```python
from build123d import *

# Parameters (mm, degrees)
ESQUISSE2_W             = 154.6
ESQUISSE2_H             = 3
BOSS_EXTRU_1_DEPTH      = 64.27
ESQUISSE3_R             = 2.5
ENL_V_MAT_EXTRU_1_DEPTH = 101.761443216
ENL_V_MAT_EXTRU_2_DEPTH = 101.761443216


with BuildPart() as part:
    # Esquisse2 → Boss.-Extru.1 (new body)
    with BuildSketch(Plane(origin=(0, 0, 0), x_dir=(1, 0, 0), z_dir=(0, 1, 0))):
        with Locations((-0.245054897, 0)):
            Rectangle(ESQUISSE2_W, ESQUISSE2_H)
    extrude(amount=BOSS_EXTRU_1_DEPTH)

    # Esquisse3 → Enlèv. mat.-Extru.1 (cut, through all)
    with BuildSketch(Plane.XY.offset(1.5)):
        with Locations((-67.545054897, 16.0675)):
            Circle(ESQUISSE3_R)
        with Locations((-67.545054897, 48.2025)):
            Circle(ESQUISSE3_R)
        with Locations((67.054945103, 48.2025)):
            Circle(ESQUISSE3_R)
        with Locations((67.054945103, 16.0675)):
            Circle(ESQUISSE3_R)
    extrude(amount=-ENL_V_MAT_EXTRU_1_DEPTH, mode=Mode.SUBTRACT)

    # Esquisse4 → Enlèv. mat.-Extru.2 (cut, through all)
    with BuildSketch(Plane.XY.offset(1.5)):
        with BuildLine():
            Line((-46.395054897, 47.135), (-46.395054897, 17.135))
            ThreePointArc((-46.395054897, 17.135), (-38.895054897, 9.635), (-31.395054897, 17.135))
            Line((-31.395054897, 17.135), (-31.395054897, 47.135))
            ThreePointArc((-31.395054897, 47.135), (-38.895054897, 54.635), (-46.395054897, 47.135))
        make_face()
        with BuildLine():
            Line((-7.745054897, 47.135), (-7.745054897, 17.135))
            ThreePointArc((-7.745054897, 17.135), (-0.245054897, 9.635), (7.254945103, 17.135))
            Line((7.254945103, 17.135), (7.254945103, 47.135))
            ThreePointArc((7.254945103, 47.135), (-0.245054897, 54.635), (-7.745054897, 47.135))
        make_face()
        with BuildLine():
            Line((30.904945103, 47.135), (30.904945103, 17.135))
            ThreePointArc((30.904945103, 17.135), (38.404945103, 9.635), (45.904945103, 17.135))
            Line((45.904945103, 17.135), (45.904945103, 47.135))
            ThreePointArc((45.904945103, 47.135), (38.404945103, 54.635), (30.904945103, 47.135))
        make_face()
    extrude(amount=-ENL_V_MAT_EXTRU_2_DEPTH, mode=Mode.SUBTRACT)


solid = part.part
```
Geometry check sheet. Reference: the model listing, model coordinates, mm. A direction names the side the tool comes from. Give positions to 0.01 mm unless a question says otherwise; leave off trailing zeros. Loops run counter-clockwise (first coordinate to the right, second up) from the corner with the lowest first, then second, coordinate; pieces in that order, holes last. Notation, with made-up numbers: M -36,66.5 L -19,66.5 A17 cw -19,74.5 Z; hole C 52.25,-26.5 d11. An arc over 180 degrees is marked long. Write item = value, one per line. Start each with the question number.
1. Draft check along Y on faces 1 (the face through (69.44, 16.82, 0.02)), 2 (the face through (30.905, 32, 0)), 3 (the face through (-1, 0, 0)), 4 (the face through (-1, 64.27, 0)). Enter one of: +Y half, -Y half, draft (parallel to the pull), parting line (faces both ways), or undercut.
2. Tool access check on faces 5 (the face through (-38.73, 54.633, 0.021)), 6 (the face through (-19, 32, 1.5)). Record the directions out of +Z, -Z, +X, -X, +Y, -Y that give a thin tool (end or side, any length) a straight path to the whole face; none if there is none.
3. Section check A-A, the plane y = 39.5. Enter the section's corners in (x, z), plus the area to 3 significant figures.
4. Go/stop test with a flat-tipped pin: P1, Ø4.5, axis at x = -67.55, y = 16.07, coming from the +Z side. Record where the tip stops, or that it passes through.
5. Section check C-C, the plane x = 5. Enter the section's corners in (y, z), plus the area to 3 significant figures.
6. Section check B-B, the plane z = -0.9. Enter the section's corners in (x, y) (1 decimal).
7. Thickness scan on probe 1 along X at (y, z) = (33.5, 1.1); probe 2 along X at (y, z) = (52.5, 0.3); probe 3 along X at (y, z) = (46, -1.1). Record the ranges inside material, lowest first.
Values follow:
q1.face_1 = undercut
q1.face_2 = undercut
q1.face_3 = -Y half
q1.face_4 = +Y half
q2.face_5 = +Z, -Z
q2.face_6 = +Z, +X, -X, +Y, -Y
q3.outline = M -77.55,-1.5 L -46.4,-1.5 L -46.4,1.5 L -77.55,1.5 Z; M -31.4,-1.5 L -7.75,-1.5 L -7.75,1.5 L -31.4,1.5 Z; M 7.25,-1.5 L 30.9,-1.5 L 30.9,1.5 L 7.25,1.5 Z; M 45.9,-1.5 L 77.05,-1.5 L 77.05,1.5 L 45.9,1.5 Z
q3.area = 329 mm^2
q4.P1 = through
q5.outline = M 0,-1.5 L 11.77,-1.5 L 11.77,1.5 L 0,1.5 Z; M 52.5,-1.5 L 64.27,-1.5 L 64.27,1.5 L 52.5,1.5 Z
q5.area = 70.6 mm^2
q6.outline = M -77.5,0 L 77.1,0 L 77.1,64.3 L -77.5,64.3 Z; hole C -67.5,16.1 d5; hole C -67.5,48.2 d5; hole M -46.4,17.1 A7.5 ccw -31.4,17.1 L -31.4,47.1 A7.5 ccw -46.4,47.1 Z; hole M -7.7,17.1 A7.5 ccw 7.3,17.1 L 7.3,47.1 A7.5 ccw -7.7,47.1 Z; hole M 30.9,17.1 A7.5 ccw 45.9,17.1 L 45.9,47.1 A7.5 ccw 30.9,47.1 Z; hole C 67.1,16.1 d5; hole C 67.1,48.2 d5
q7.probe_1 = -77.55 to -46.4, -31.4 to -7.75, 7.25 to 30.9, 45.9 to 77.05
q7.probe_2 = -77.55 to -44.14, -33.65 to -5.49, 5 to 33.16, 43.65 to 77.05
q7.probe_3 = -77.55 to -68.73, -66.36 to -46.4, -31.4 to -7.75, 7.25 to 30.9, 45.9 to 65.87, 68.24 to 77.05
